Input: part model. Units: mm. Frame: model coordinates. A direction names the side the tool comes from. Give positions to 0.01 mm unless a question says otherwise; leave off trailing zeros. Loops run counter-clockwise (first coordinate to the right, second up) from the corner with the lowest first, then second, coordinate; pieces in that order, holes last. Notation, with made-up numbers: (-21.5, -15) - (31.5, -15) arc R25 ccw to (31.5, 12) - close; hole circle Ø8 at (52, 55). An arc over 180 degrees is marked (long way). Answer as a JSON object with one key per item and string values. Group by question number.
(1) Material intervals for L1, parallel to Z at x = 10.5, y = 24 (3 decimals); L2, parallel to Y at x = 18, z = 8; L3, parallel to X at y = 4, z = -3.5, sorted ascending.
(2) Section query C-C (z = -7.5). Return loops of the section in (x, y).
(3) Mould query, pull axis Z, two halves, no side actions, for faces 5 (the cylindrical face through (18, 3.8, 6.8)), 6 (the flat face through (16.5, 3, 0)), 7 (the flat face through (-11, 15, -21)), 8 (the flat face through (0, 9, -22.775)). Classes: +Z half, -Z half, draft (parallel to the pull), parting line (faces both ways), or undercut.
(4) Pin query (flat end, axial travel): P1, Ø4, axis at x = -13, z = 2, coming from the +Y side; P2, Ø2.5, axis at y = 17, z = -21, coming from the -X side; P3, Ø0.9, axis at y = 21, z = 22, coming from the +X side; P4, Ø1.3, axis at x = -5.66, y = 13.34, coming from the +Z side (3 decimals). Return the tip coordinate at first contact, or that it passes through.
(5) Section query D-D (z = -17). Return loops of the section in (x, y).
(6) Section query B-B (y = 3.3). Return loops of the section in (x, z) (3 decimals), plus the area to 3 significant figures.
(7) Access query for faces 1 (the flat face through (-17, 6, 0)), 2 (the flat face through (11, 15, -21)), 3 (the flat face through (-19.5, 3, 0)), 4 (the cylindrical face through (-6.4, 23.846, 21.296)). Directions: +Z, -Z, +X, -X, +Y, -Y. A direction counts if a zero-diameter tool reaches every point of the face in a straight line with its end or side. Return the directions, or none.
(8) Section query A-A (x = 8). Return loops of the section in (y, z) (3 decimals).
```python
from build123d import *

# Parameters (mm, degrees)
BOSS_EXTRUDE1_DEPTH   = 6
BOSS_EXTRUDE1_2_DEPTH = 6
SKETCH1_3_W           = 22
SKETCH1_3_H           = 3
BOSS_EXTRUDE2_DEPTH   = 30
SKETCH1_4_W           = 22
SKETCH1_4_H           = 3
BOSS_EXTRUDE3_DEPTH   = 24.4
CUT_EXTRUDE1_REACH    = 56.219
SKETCH3_R             = 1.3
SKETCH4_R             = 1.6
CUT_EXTRUDE2_DEPTH    = 3
SKETCH5_R             = 3
SKETCH5_R_2           = 1.1
CUT_EXTRUDE3_DEPTH    = 3
CIRPATTERN1_COUNT     = 4


with BuildPart() as part:
    # Sketch1 → Boss-Extrude1 (new body)
    with BuildSketch(Plane(origin=(0, 0, 0), x_dir=(1, 0, 0), z_dir=(0, 1, 0))):
        Polygon((-11, 19.775), (-11, 22.775), (-19.5, 22.775), (-19.5, -22.775), (-11, -22.775), (-11, -19.775), (-16.5, -19.775), (-16.5, 19.775), align=None)
    extrude(amount=BOSS_EXTRUDE1_DEPTH)



with BuildPart() as body_2:
    # Sketch1 → Boss-Extrude1 2 (new body)
    with BuildSketch(Plane(origin=(0, 0, 0), x_dir=(1, 0, 0), z_dir=(0, 1, 0))):
        Polygon((19.5, -22.775), (19.5, 22.775), (11, 22.775), (11, 19.775), (16.5, 19.775), (16.5, -19.775), (11, -19.775), (11, -22.775), align=None)
    extrude(amount=BOSS_EXTRUDE1_2_DEPTH)


with BuildPart() as part_1:
    add(part.part)

    add(body_2.part)  # Boss-Extrude2 merges body 2
    # Sketch1<3> → Boss-Extrude2 (add)
    with BuildSketch(Plane(origin=(0, 0, 0), x_dir=(1, 0, 0), z_dir=(0, 1, 0))):
        with Locations((0, -21.275)):
            Rectangle(SKETCH1_3_W, SKETCH1_3_H)
    extrude(amount=BOSS_EXTRUDE2_DEPTH)

    # Sketch1<4> → Boss-Extrude3 (add)
    with BuildSketch(Plane(origin=(0, 0, 0), x_dir=(1, 0, 0), z_dir=(0, 1, 0))):
        with Locations((0, 21.275)):
            Rectangle(SKETCH1_4_W, SKETCH1_4_H)
    extrude(amount=BOSS_EXTRUDE3_DEPTH)

    # Cut-Extrude1: up to this face of the body (flat: up to its plane)
    cut_extrude1_end = Plane(part_1.part.faces().sort_by_distance((19.5, 3, 0))[0])
    # Sketch3 → Cut-Extrude1 (cut, up to the picked face)
    with BuildSketch(Plane.ZY.offset(19.5), mode=Mode.PRIVATE) as cut_extrude1_sk1:
        with Locations((-8, 3.3)):
            Circle(SKETCH3_R)
    cut_extrude1_tool1 = split(extrude(cut_extrude1_sk1.sketch, amount=-CUT_EXTRUDE1_REACH, mode=Mode.PRIVATE), bisect_by=cut_extrude1_end, keep=Keep.BOTH, mode=Mode.PRIVATE)
    # Sketch3 → Cut-Extrude1 (cut, up to the picked face)
    with BuildSketch(Plane.ZY.offset(19.5), mode=Mode.PRIVATE) as cut_extrude1_sk2:
        with Locations(Location((8, 3.3, 0), (0, 0, 180))):
            Circle(SKETCH3_R)
    cut_extrude1_tool2 = split(extrude(cut_extrude1_sk2.sketch, amount=-CUT_EXTRUDE1_REACH, mode=Mode.PRIVATE), bisect_by=cut_extrude1_end, keep=Keep.BOTH, mode=Mode.PRIVATE)
    add(cut_extrude1_tool1.solids().sort_by(Axis((-19.5, 3.3, -8), (1, 0, 0)))[0], mode=Mode.SUBTRACT)
    add(cut_extrude1_tool2.solids().sort_by(Axis((-19.5, 3.3, 8), (1, 0, 0)))[0], mode=Mode.SUBTRACT)

    # Sketch4 → Cut-Extrude2 (cut)
    with BuildSketch(Plane(origin=(0, 0, -22.775), x_dir=(-1, 0, 0), z_dir=(0, 0, -1))):
        with Locations((0, 19)):
            Circle(SKETCH4_R)
    extrude(amount=-CUT_EXTRUDE2_DEPTH, mode=Mode.SUBTRACT)

    # Sketch5 → Cut-Extrude3 (cut)
    with BuildSketch(Plane.XY.offset(22.775)):
        with Locations((0, 19)):
            Circle(SKETCH5_R)
        with Locations((5.656854249, 24.656854249)):
            Circle(SKETCH5_R_2)
    cut_extrude3 = extrude(amount=-CUT_EXTRUDE3_DEPTH, mode=Mode.SUBTRACT)

    # CirPattern1: Cut-Extrude3 ×4 about axis
    cirpattern1_axis = Axis((0, 19, 0), (0, 0, 1))
    for i in range(1, CIRPATTERN1_COUNT):
        add(cut_extrude3.rotate(cirpattern1_axis, i * 360 / CIRPATTERN1_COUNT), mode=Mode.SUBTRACT)


solid = part_1.part
```
Recorded:
{
 "1": {"L1": "z = -22.775 to -19.775, 19.775 to 22.775", "L2": "y = 0 to 2, 4.6 to 6", "L3": "x = -19.5 to -16.5, 16.5 to 19.5"},
 "2": {"outline": "(-19.5, 0) - (-16.5, 0) - (-16.5, 2.1) - (-19.5, 2.1) - close; (-19.5, 4.5) - (-16.5, 4.5) - (-16.5, 6) - (-19.5, 6) - close; (16.5, 0) - (19.5, 0) - (19.5, 2.1) - (16.5, 2.1) - close; (16.5, 4.5) - (19.5, 4.5) - (19.5, 6) - (16.5, 6) - close"},
 "3": {"face 5": "undercut", "face 6": "undercut", "face 7": "draft", "face 8": "-Z half"},
 "4": {"P1": "passes through", "P2": "stops at x = -11", "P3": "stops at x = 11", "P4": "stops at z = -19.775"},
 "5": {"outline": "(-19.5, 0) - (-16.5, 0) - (-16.5, 6) - (-19.5, 6) - close; (16.5, 0) - (19.5, 0) - (19.5, 6) - (16.5, 6) - close"},
 "6": {"outline": "(-19.5, -22.775) - (19.5, -22.775) - (19.5, -9.3) - (16.5, -9.3) - (16.5, -19.775) - (-16.5, -19.775) - (-16.5, -9.3) - (-19.5, -9.3) - close; (-19.5, -6.7) - (-16.5, -6.7) - (-16.5, 6.7) - (-19.5, 6.7) - close; (-19.5, 9.3) - (-16.5, 9.3) - (-16.5, 19.775) - (16.5, 19.775) - (16.5, 9.3) - (19.5, 9.3) - (19.5, 22.775) - (-19.5, 22.775) - close; (16.5, -6.7) - (19.5, -6.7) - (19.5, 6.7) - (16.5, 6.7) - close", "area": "440 mm^2"},
 "7": {"face 1": "+Z, -Z, -X, +Y", "face 2": "+Z, -Z, +X, +Y", "face 3": "+Z, -Z, -X, +Y, -Y", "face 4": "+Z"},
 "8": {"outline": "(0, -22.775) - (24.4, -22.775) - (24.4, -19.775) - (0, -19.775) - close; (0, 19.775) - (30, 19.775) - (30, 22.775) - (0, 22.775) - close"}
}
